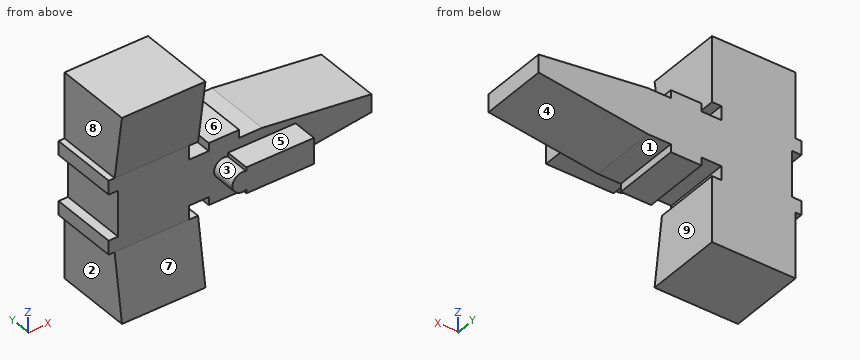
from build123d import *

# Parameters (mm, degrees)
BOSS_EXTRUDE1_DEPTH = 17
BOSS_EXTRUDE2_DEPTH = 6.25
BOSS_EXTRUDE3_DEPTH = 21


with BuildPart() as part:
    # Sketch1 → Boss-Extrude1 (new body)
    with BuildSketch(Plane(origin=(0, 0, 0), x_dir=(1, 0, 0), z_dir=(0, 1, 0))):
        Polygon((38.887869235, 32.64650928), (33.855356453, 32.64650928), (33.855356453, 36.14650928), (36.187130568, 36.14650928), (36.187130568, 52.64650928), (15.187130568, 52.64650928), (15.187130568, 36.14650928), (13.687130568, 36.14650928), (13.687130568, 32.64650928), (16.05811547, 32.64650928), (16.05811547, 21.14650928), (13.687130568, 21.14650928), (13.687130568, 17.64650928), (15.187130568, 17.64650928), (15.187130568, 1.14650928), (36.187130568, 1.14650928), (36.187130568, 17.64650928), (33.855356453, 17.64650928), (33.855356453, 21.14650928), (38.887869235, 21.14650928), (38.887869235, 19.14650928), (46.537869235, 19.14650928), (46.537869235, 21.14650928), (52.287869235, 21.14650928), (79.808081842, 24.64650928), (79.808081842, 29.14650928), (52.287869235, 32.64650928), (46.537869235, 32.64650928), (46.537869235, 34.64650928), (38.887869235, 34.64650928), align=None)
    extrude(amount=BOSS_EXTRUDE1_DEPTH)

    # Sketch2 → Boss-Extrude2 (add)
    with BuildSketch(Plane.XZ):
        with BuildLine():
            Line((43.712869235, -29.187797128), (43.712869235, -30.14650928))
            Line((43.712869235, -30.14650928), (45.212869235, -30.14650928))
            Line((45.212869235, -30.14650928), (60.712869235, -30.14650928))
            Line((60.712869235, -30.14650928), (60.712869235, -26.89650928))
            Line((60.712869235, -26.89650928), (60.712869235, -23.64650928))
            Line((60.712869235, -23.64650928), (45.212869235, -23.64650928))
            Line((45.212869235, -23.64650928), (43.712869235, -23.64650928))
            Line((43.712869235, -23.64650928), (43.712869235, -24.605221433))
            ThreePointArc((43.712869235, -24.605221433), (40.212869235, -26.89650928), (43.712869235, -29.187797128))
        make_face()
    extrude(amount=BOSS_EXTRUDE2_DEPTH)

    # Sketch3 → Boss-Extrude3 (add)
    with BuildSketch(Plane.ZY.offset(-15.187130568)):
        Polygon((-1.14650928, 0), (-1.14650928, -2.5), (-17.64650928, 0), align=None)
        Polygon((-36.14650928, 0), (-52.64650928, 0), (-52.64650928, -2.5), align=None)
    extrude(amount=-BOSS_EXTRUDE3_DEPTH)


solid = part.part
Design review of the part built by this model. Coordinates are the model's own, in mm. Face numbers are marked on the shaded views. A direction names the side the tool comes from. Coordinates: 2 decimals unless noted, no trailing zeros. Order: outer loops, then holes, each group sorted by start corner. A loop starts at its lowest first (then second) coordinate and runs counter-clockwise, first axis right, second up. Notation, with made-up numbers: (-39, 12.25) - (9, 12.25) arc R31 ccw to (9, 46.25) - close; hole circle Ø6 at (63, 19.5). An arc over 180 degrees is marked (long way). Put each result on its own line as item: value.
1) Wall thickness on L1, parallel to X at y = 1.75, z = -21; L2, parallel to Z at x = 34.5, y = 8.25; L3, parallel to Y at x = 20.5, z = -19: over which ranges is each line inside the solid? List them lowest first. Write a range as from..to.
Response values:
L1: x = 13.69..33.86, 38.89..46.54
L2: z = -52.65..-36.15, -32.65..-21.15, -17.65..-1.15
L3: y = 0..17
2) Take a section at B-B, the plane x = 21. Give the boundary of the cut face in (y, z), and give its area (3 significant figures).
Response values:
outline: (-2.5, -52.65) - (17, -52.65) - (17, -1.15) - (-2.5, -1.15) - (0, -17.65) - (0, -36.15) - close
area: 917 mm²
3) Take a section at C-C, the plane y = -1.75. Give the boundary of the cut face in (x, z).
Response values:
outline: (15.19, -52.65) - (36.19, -52.65) - (36.19, -47.7) - (15.19, -47.7) - close; (15.19, -6.1) - (36.19, -6.1) - (36.19, -1.15) - (15.19, -1.15) - close; (43.71, -30.15) - (60.71, -30.15) - (60.71, -23.65) - (43.71, -23.65) - (43.71, -24.61) arc R2.5 ccw (long way) to (43.71, -29.19) - close
4) The part is to be moulded in two halves that separate along X. For the marked faces 1, 2, 3 and 4, say which applies: released by +X, released by -X, zero draft, split by the parting line, or undercut.
Response values:
face 1: zero draft
face 2: released by -X
face 3: undercut
face 4: released by +X
5) Take a section at D-D, the plane x = 47.5. Give the boundary of the cut face in (y, z).
Response values:
outline: (-6.25, -30.15) - (0, -30.15) - (0, -32.65) - (17, -32.65) - (17, -21.15) - (0, -21.15) - (0, -23.65) - (-6.25, -23.65) - close
6) Insertion check: P1, Ø0.8, axis at x = 14.5, y = 9, coming from the -Z side; P2, Ø6.5, axis at x = 50.5, y = 5, coming from the -Z side; P3, Ø10, axis at x = 34.5, z = -10.5, coming from the -Y side. Each pin has a flat end and moves straight along its axis. Give the tip position at first contact, or say it passes through.
Response values:
P1: stops at z = -36.15
P2: stops at z = -32.65
P3: stops at y = -1.84
7) Tool access review of the marked faces 5, 6, 7, 8 and 9: name each direction out of +Z, -Z, +X, -X, +Y, -Y from which nothing blocks a thin tool from reaching the whole face with its end or side.
Response values:
face 5: +Z, +X, -X, -Y
face 6: +Z, +X, +Y, -Y
face 7: +X, -X, -Y
face 8: +Z, -X, +Y, -Y
face 9: -Z, +X, +Y, -Y
